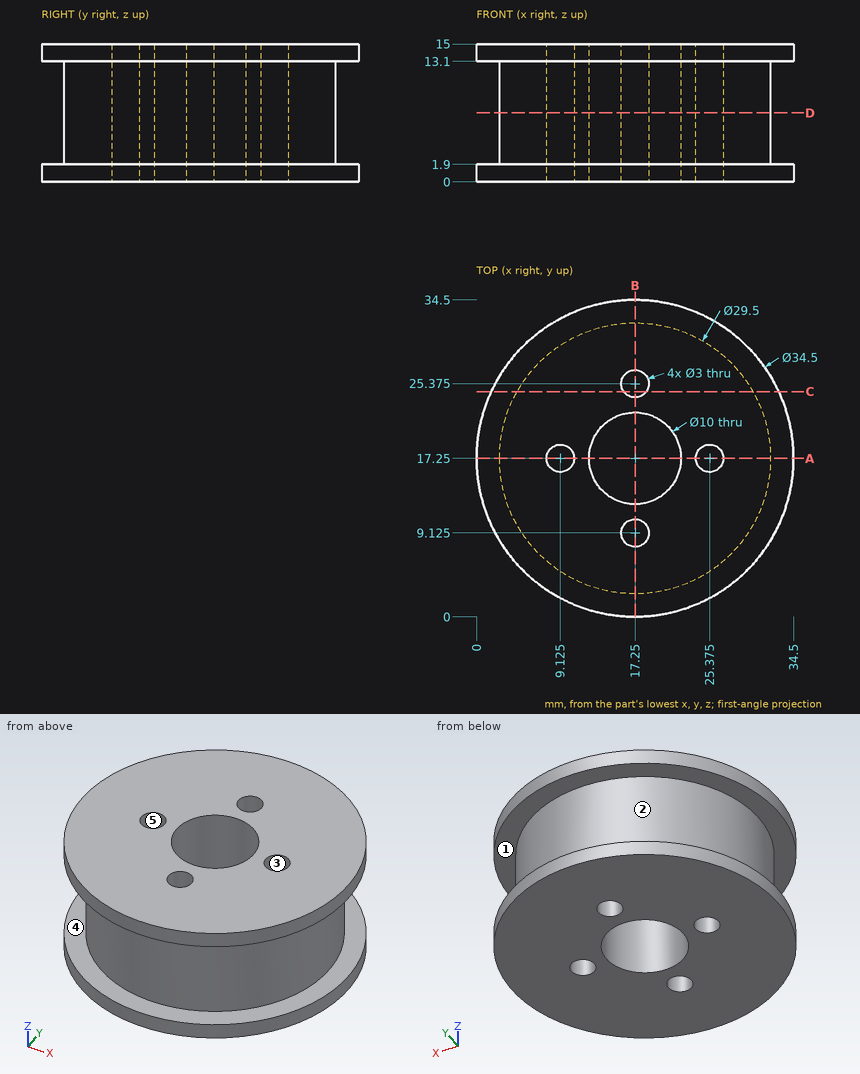
Input: dimensioned drawing with shaded views. Units: mm. Origin: part minimum x, y, z. A direction names the side the tool comes from. Coordinates: 2 decimals unless noted, no trailing zeros. Order: outer loops, then holes, each group sorted by start corner. A loop starts at its lowest first (then second) coordinate and runs counter-clockwise, first axis right, second up. Notation, with made-up numbers: M 44.25,-32.75 L 55.25,-32.75 A24 ccw 55.25,4.25 Z; hole C 28,62.5 d2. An arc over 180 degrees is marked long. Answer as CSV lines item,"result".
Q1. First-contact query: P1, Ø2.5, axis at x = 9.125, y = 17.25, coming from the -Z side; P2, Ø3, axis at y = 17, z = 7.5, coming from the -X side; P3, Ø4, axis at x = 5, z = 12.5, coming from the +Y side; P4, Ø2, axis at x = 7, z = 2.5, coming from the -Y side. Flat tips, straight axial feed; report the tip coordinate or a pass-through.
Answers:
P1,"passes through"
P2,"stops at x = 2.5"
P3,"stops at y = 31.06"
P4,"stops at y = 2.82"
Q2. Draft query along Y for the marked faces 1, 2 and 3. Return one class per face: pulls with the +Y half, pulls with the -Y half, needs draft (parallel to the pull), parting line crosses it, or undercut.
Answers:
face 1,"needs draft"
face 2,"parting line crosses it"
face 3,"undercut"
Q3. Line query: probe 1 along Y at (x, z) = (17.25, 4.5) (3 decimals); probe 2 along Z at (x, y) = (10.5, 2.5); probe 3 along X at (y, z) = (17, 12.75). Output: solid intervals per line, ascending. Write a range as [from, to].
Answers:
probe 1,"y = [2.5, 7.625], [10.625, 12.25], [22.25, 23.875], [26.875, 32]"
probe 2,"z = [0, 1.9], [13.1, 15]"
probe 3,"x = [2.5, 7.65], [10.6, 12.26], [22.24, 23.9], [26.85, 32]"
Q4. Section D-D on z = 7.5. Return the cut outline in (x, y) (3 decimals), and give its area (3 significant figures).
Answers:
outline,"C 17.25,17.25 d29.5; hole C 9.125,17.25 d3; hole C 17.25,17.25 d10; hole C 17.25,9.125 d3; hole C 17.25,25.375 d3; hole C 25.375,17.25 d3"
area,"577 mm^2"
Q5. Set-up query: the marked faces 4 and 5. Return all of +Z, -Z, +X, -X, +Y, -Y with unobstructed straight access to the full face (end or side cutting, diameter ignored); none if empty.
Answers:
face 4,"none"
face 5,"+Z, -Z"
Q6. Section C-C on y = 24.5. Return the cut outline in (x, z), and give its area (3 significant figures).
Answers:
outline,"M 1.6,0 L 16.03,0 L 16.03,15 L 1.6,15 L 1.6,13.1 L 4.4,13.1 L 4.4,1.9 L 1.6,1.9 Z; M 18.47,0 L 32.9,0 L 32.9,1.9 L 30.1,1.9 L 30.1,13.1 L 32.9,13.1 L 32.9,15 L 18.47,15 Z"
area,"370 mm^2"
Q7. Section A-A on y = 17.25. Return the cut outline in (x, z) (3 decimals).
Answers:
outline,"M 0,0 L 7.625,0 L 7.625,15 L 0,15 L 0,13.1 L 2.5,13.1 L 2.5,1.9 L 0,1.9 Z; M 10.625,0 L 12.25,0 L 12.25,15 L 10.625,15 Z; M 22.25,0 L 23.875,0 L 23.875,15 L 22.25,15 Z; M 26.875,0 L 34.5,0 L 34.5,1.9 L 32,1.9 L 32,13.1 L 34.5,13.1 L 34.5,15 L 26.875,15 Z"
